Verification items for the finished model (mm, model axes). Give positions to 0.01 mm unless a question says otherwise; leave off trailing zeros. Order: outer loops, then holes, each group sorted by start corner. A loop starts at its lowest first (then second) coordinate and runs counter-clockwise, first axis right, second up. Notation, with made-up numbers: (15, -25.75) - (19, -25.75) arc R23 cw to (19, -3.75) - close; hole circle Ø4 at (0.5, 23.25). An arc over 180 degrees is marked (long way). Answer as a JSON object with one key per item and string values. Group by question number.
(1) Mould release check, pull along X, two halves, no side actions. Record for faces 1 (the face through (-1.2, 0, -1.2)), 2 (the face through (-0.867, 1.913, 3.905)), 3 (the face through (-1.5, 1.55, -0.07)): +X half, -X half, draft (parallel to the pull), parting line (faces both ways), or undercut.
(2) Thickness scan on line 1 (X direction, y = 2, z = 0); line 2 (Z direction, x = 0, y = 0.75). Record the ranges inside material, lowest first.
(3) Section check B-B (z = 0). Record the boundary of the cut face in (x, y).
(4) Depth check by flat-ended pin: pin 1 Ø1.5 at (x, y) = (2, 2) entering from +Z; pin 2 Ø1 at (y, z) = (1, -3) entering from -X. Enter the tip coordinate at first touch or a pass-through.
(5) Section check D-D (z = -4.5). Record the boundary of the cut face in (x, y), then the cut area to 3 significant figures.
(6) Section check A-A (x = 0). Record the boundary of the cut face in (y, z).
(7) Section check C-C (y = 1.3). Record the boundary of the cut face in (x, z), then the cut area to 3 significant figures.
```python
from build123d import *

# Parameters (mm, degrees)
SKETCH1_R           = 5
BOSS_EXTRUDE1_DEPTH = 1.05
SKETCH2_R           = 4
BOSS_EXTRUDE2_DEPTH = 2
SKETCH3_R           = 1.5
CUT_EXTRUDE1_DEPTH  = 12
CHAMFER2_SIZE       = 0.25


with BuildPart() as part:
    # Sketch1 → Boss-Extrude1 (new body)
    with BuildSketch(Plane(origin=(0, 0, 0), x_dir=(1, 0, 0), z_dir=(0, 1, 0))):
        Circle(SKETCH1_R)
    extrude(amount=BOSS_EXTRUDE1_DEPTH)

    # Sketch2 → Boss-Extrude2 (add)
    with BuildSketch(Plane(origin=(0, 1.05, 0), x_dir=(1, 0, 0), z_dir=(0, 1, 0))):
        Circle(SKETCH2_R)
    extrude(amount=BOSS_EXTRUDE2_DEPTH)

    # Sketch3 → Cut-Extrude1 (cut)
    with BuildSketch(Plane(origin=(0, 3.05, 0), x_dir=(1, 0, 0), z_dir=(0, 1, 0))):
        Circle(SKETCH3_R)
    extrude(amount=-CUT_EXTRUDE1_DEPTH, mode=Mode.SUBTRACT)

    # Chamfer2
    chamfer2_edges = [part.edges().sort_by_distance(p)[0] for p in [
        (-4, 3.05, 0),
    ]]
    chamfer(chamfer2_edges, length=CHAMFER2_SIZE)


solid = part.part
```
Solutions:
{
 "1": {"face 1": "draft", "face 2": "parting line", "face 3": "undercut"},
 "2": {"line 1": "x = -4 to -1.5, 1.5 to 4", "line 2": "z = -5 to -1.5, 1.5 to 5"},
 "3": {"outline": "(-5, 0) - (-1.5, 0) - (-1.5, 3.05) - (-3.75, 3.05) - (-4, 2.8) - (-4, 1.05) - (-5, 1.05) - close; (1.5, 0) - (5, 0) - (5, 1.05) - (4, 1.05) - (4, 2.8) - (3.75, 3.05) - (1.5, 3.05) - close"},
 "4": {"pin 1": "stops at z = 3.8", "pin 2": "stops at x = -4.33"},
 "5": {"outline": "(-2.18, 0) - (2.18, 0) - (2.18, 1.05) - (-2.18, 1.05) - close", "area": "4.58 mm2"},
 "6": {"outline": "(0, -5) - (1.05, -5) - (1.05, -4) - (2.8, -4) - (3.05, -3.75) - (3.05, -1.5) - (0, -1.5) - close; (0, 1.5) - (3.05, 1.5) - (3.05, 3.75) - (2.8, 4) - (1.05, 4) - (1.05, 5) - (0, 5) - close"},
 "7": {"outline": "circle Ø8 at (0, 0); hole circle Ø3 at (0, 0)", "area": "43.2 mm2"}
}
